Source: three-view drawing plus pictorial views. Frame: mm from the lowest corner of the part. Give positions to 0.01 mm unless a question says otherwise; leave off trailing zeros. Order: outer loops, then holes, each group sorted by start corner. A loop starts at its lowest first (then second) coordinate and runs counter-clockwise, first axis right, second up. Notation, with made-up numbers: (84.25, -17) -> (138.25, -17) arc R17 ccw to (138.25, -12) -> close; hole circle Ø8 at (73, 79.5). An arc over 180 degrees is marked (long way). One line per question, with ' | ' between items.
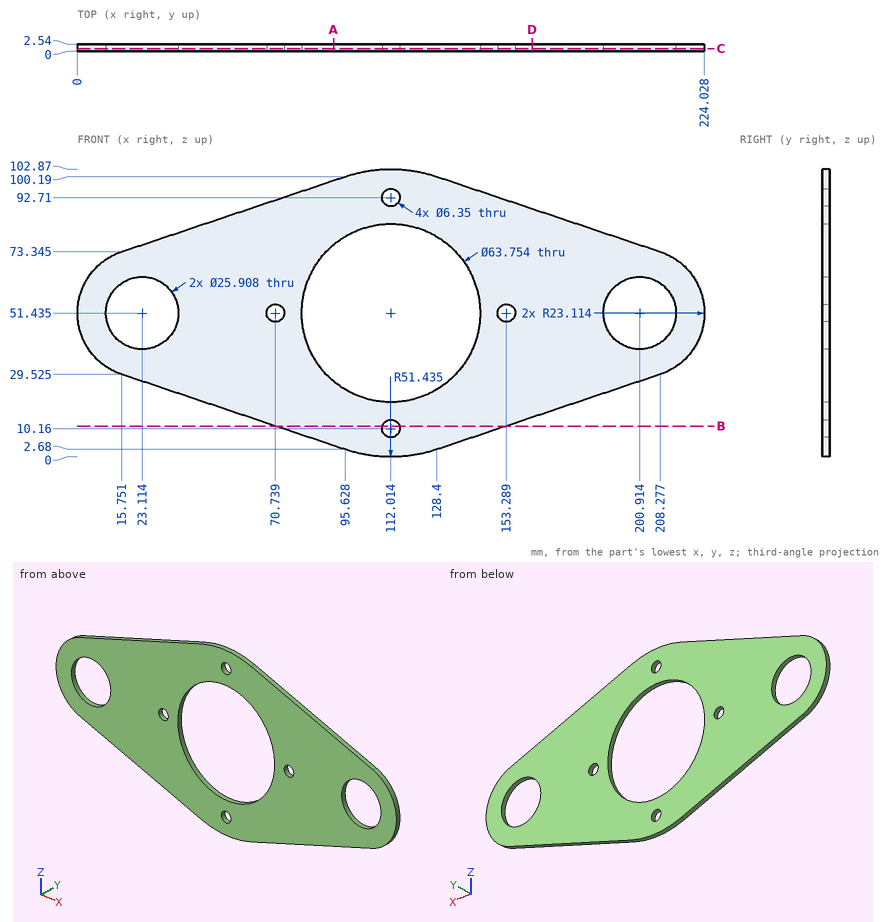
1) Section D-D on x = 162.5. Return loops of the section in (y, z).
Check result:
outline: (0, 14.14) -> (2.54, 14.14) -> (2.54, 88.73) -> (0, 88.73) -> close
2) Contact query for a flat-ended pin moving along its axis: pin 1 Ø23.5 at (x, z) = (23.114, 51.435) entering from +Y. Output: stop coordinate, or through.
Check result:
pin 1: passes through
3) Section A-A on x = 91.5. Return loops of the section in (y, z) (1 decimal), plus the area to 3 significant figures.
Check result:
outline: (0, 4.1) -> (2.5, 4.1) -> (2.5, 27) -> (0, 27) -> close; (0, 75.8) -> (2.5, 75.8) -> (2.5, 98.8) -> (0, 98.8) -> close | area: 117 mm^2
4) Section B-B on z = 11. Return loops of the section in (x, y) (1 decimal).
Check result:
outline: (70.9, 0) -> (109, 0) -> (109, 2.5) -> (70.9, 2.5) -> close; (115.1, 0) -> (153.2, 0) -> (153.2, 2.5) -> (115.1, 2.5) -> close
5) Material intervals for probe 1 along X at (y, z) = (1.05, 56) (1 decimal); probe 2 along X at (y, z) = (1.65, 44) (1 decimal); probe 3 along Z at (x, y) = (200.5, 0.8), sorted ascending. Write a range as from..to.
Check result:
probe 1: x = 0.5..11, 35.2..80.5, 143.6..188.8, 213..223.6 | probe 2: x = 1.2..12.5, 33.7..81, 143..190.3, 211.5..222.8 | probe 3: z = 26.91..38.49, 64.38..75.96
6) Section C-C on y = 0.9. Count the separate pieces of the cut face and the enclosed holes in it, plus the area to 3 significant figures.
Check result:
separate pieces: 1 | enclosed holes: 7 | area: 11,200 mm^2
